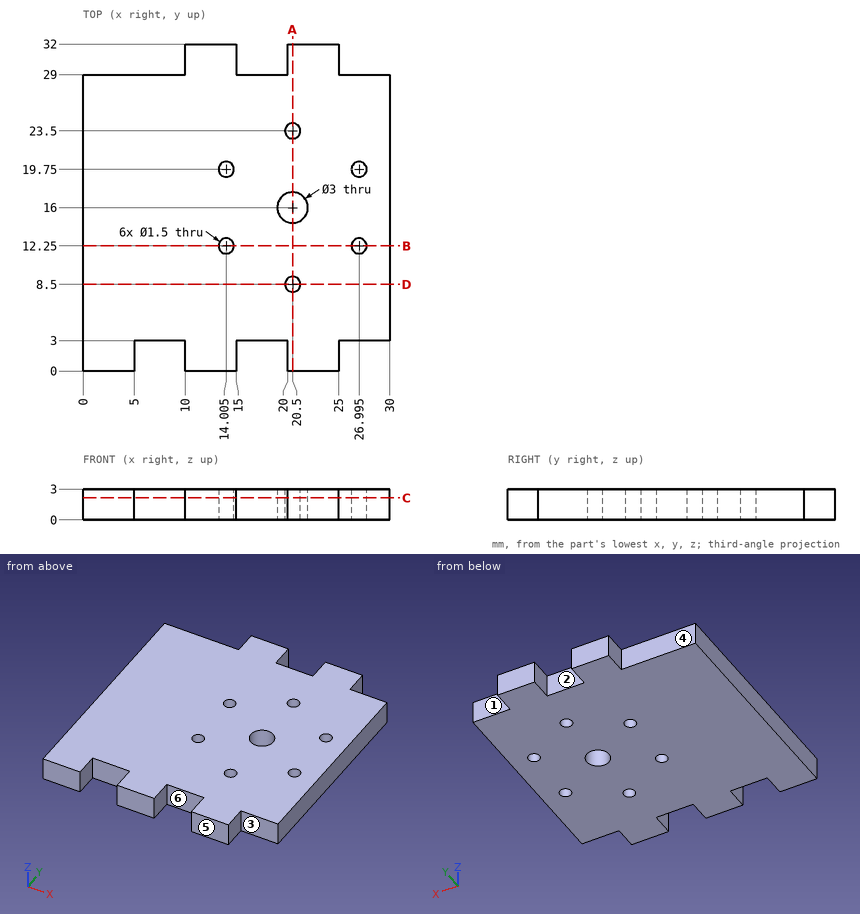
Drawing for the job (mm, zero at the part's lowest x, y, z). A direction names the side the tool comes from. Round coordinates to 2 decimals unless told otherwise and drop trailing zeros. Write each loop counter-clockwise with the first axis right and the second up, starting at its lowest first coordinate (ties: lowest second). Pieces come first, ordered by that corner, then holes. Notation, with made-up numbers: (47.5, 18.5) - (62.5, 18.5) arc R38 cw to (62.5, 57.5) - close; hole circle Ø4 at (40.5, 68). An arc over 180 degrees is marked (long way). Write item = value, one per line. Start each with the question number.
Q1. Band-saw the part on C-C (z = 2.15). Count the separate pieces of the cut face and the enclosed holes in it, then the cut area to 3 significant figures.
Q2. Drop flat-ended pins along their axis: pin 1 (2 mm diameter, centred on x = 14, y = 19.75, fed in from +Z); pin 2 (0.9 mm diameter, centred on x = 6.5, z = 1, fed in from -Y); pin 3 (0.9 mm diameter, centred on y = 30.5, z = 1.5, fed in from -X); pin 4 (0.9 mm diameter, centred on x = 4.5, z = 2, fed in from +Y). Give the stop position or say it passes through.
Q3. Probe L1, parallel to Y at x = 20.5, z = 2.4; L2, parallel to Y at x = 27, z = 1.9; L3, parallel to Y at x = 14.25, z = 0.2. List the from-to ranges inside material, lowest first. Write a range as from..to.
Q4. Mould opens along X. For the marked faces 5 and 6 say: pulls with the +X half, pulls with the -X half, needs draft (parallel to the pull), parting line crosses it, or undercut.
Q5. Band-saw the part on D-D (y = 8.5). Give the cut face in (x, z).
Q6. Band-saw the part on A-A (x = 20.5). Give the cut face in (y, z), then the cut area to 3 significant figures.
Q7. Which spindle directions (+Z, -Z, +X, -X, +Y, -Y) get a long thin tool onto all of the face, cutting with end or side? Do the marked faces 1, 2, 3 and 4. Say none if no direction does.
Q8. Band-saw the part on B-B (y = 12.25). Give the cut face in (x, z) (1 decimal), then the cut area to 3 significant figures.
Answers below:
q1.separate_pieces = 1
q1.enclosed_holes = 7
q1.area = 837 mm2
q2.pin_1 = 3
q2.pin_2 = 3
q2.pin_3 = 10
q2.pin_4 = 29
q3.L1 = 0..7.75, 9.25..14.5, 17.5..22.75, 24.25..32
q3.L2 = 3..11.5, 13..19, 20.5..29
q3.L3 = 0..11.54, 12.96..19.04, 20.46..32
q4.face_5 = needs draft
q4.face_6 = undercut
q5.outline = (0, 0) - (19.75, 0) - (19.75, 3) - (0, 3) - close; (21.25, 0) - (30, 0) - (30, 3) - (21.25, 3) - close
q6.outline = (0, 0) - (7.75, 0) - (7.75, 3) - (0, 3) - close; (9.25, 0) - (14.5, 0) - (14.5, 3) - (9.25, 3) - close; (17.5, 0) - (22.75, 0) - (22.75, 3) - (17.5, 3) - close; (24.25, 0) - (32, 0) - (32, 3) - (24.25, 3) - close
q6.area = 78.0 mm2
q7.face_1 = +Z, -Z, +X, +Y
q7.face_2 = +Z, -Z, +Y
q7.face_3 = +Z, -Z, +X, -Y
q7.face_4 = +Z, -Z, -X, +Y
q8.outline = (0, 0) - (13.3, 0) - (13.3, 3) - (0, 3) - close; (14.8, 0) - (26.2, 0) - (26.2, 3) - (14.8, 3) - close; (27.7, 0) - (30, 0) - (30, 3) - (27.7, 3) - close
q8.area = 81.0 mm2
